Read the model definition and answer for the solid it produces. Units are mm, in the model's axes. Face numbers are marked on the shaded views. A direction names the side the tool comes from. Coordinates: 2 decimals unless noted, no trailing zeros. Write each loop counter-clockwise with the first axis right and the second up, starting at its lowest first coordinate (ties: lowest second). Pieces come first, ordered by that corner, then holes. Notation, with made-up numbers: (-28, -15) -> (-24, -15) arc R25 ccw to (-24, 24) -> close; hole circle Ø8 at (57, 63.25). An arc over 180 degrees is marked (long way). Answer in a Markdown table with one row per item. Add a question column.
Item 1: Straight lines are drawn through the part: line 1 (Y direction, x = 5.75, z = 0); line 2 (Y direction, x = 31.5, z = 5.25); line 3 (Z direction, x = 24, y = -5.5). For each, find the intervals that lie inside material, in ascending order. Write a range as from..to.
Item 2: Section B-B on z = 0 is taken. Write down the section's boundary in (x, y).
Item 3: Section C-C on x = 47.5 is taken. Write down the section's boundary in (y, z) (1 decimal), then the cut area to 3 significant figures.
Item 4: Given pin 1 Ø3 at (x, y) = (51, 1.5) entering from +Z; pin 2 Ø0.6 at (y, z) = (1.5, 4.5) entering from +X; pin 3 Ø1.5 at (x, y) = (61, -1.5) entering from -Z, each flat-ended and moving along its own axis, determine where each tip first touches the part or whether it passes through.
Item 5: Which of the six approach directions +Z, -Z, +X, -X, +Y, -Y give full straight-line access (tool end or side, diameter ignored) to the marked faces 1, 2 and 3?
Autodesk Inventor part; units mm, degrees
ref_plane "Work Plane1" through (56.23, 0, 0) normal (1, 0, 0) x (0, 0, -1)
ref_plane "YZ Plane" through (0, 0, 0) normal (1, 0, 0) x (0, 1, 0)
ref_plane "XZ Plane" through (0, 0, 0) normal (0, 1, 0) x (-1, 0, 0)
sketch "Sketch1" plane through (0, 0, 0) normal (1, 0, 0) x (0, 1, 0)
  circle A0 centre (0, 0) radius 6.35
  line L0 (0, 0) -> (0, 6.35) construction
  line L1 (-1.5875, 6.1484) -> (-1.5875, 4.7625)
  line L2 (-1.5875, 4.7625) -> (1.5875, 4.7625)
  line L3 (1.5875, 4.7625) -> (1.5875, 6.1484)
  point P0 (0, 4.7625)
  dimension "d0" = 12.7
  dimension "d2" = 1.5875
  dimension "d3" = 3.175
extrude "Extrusion1" add sketch "Sketch1" along normal blind 38.1
sketch "Sketch2" plane through (38.1, 0, 0) normal (1, 0, 0) x (0, 0, -1)
  circle A0 centre (0, 0) radius 6.35
  circle A1 centre (0, 0) radius 4.7625
  dimension "d6" = 9.525
extrude "Extrusion2" add sketch "Sketch2" along normal blind 24.13 contours A1
extrude "Extrusion3" cut sketch "Sketch1" along normal blind 34.925 contours L3 L2 L1 A0 picked at (0.1781, 5.2842)
fillet "Fillet1" radius 1.5875 2 edges at (34.925, 1.5875, 5.4554) (34.925, -1.5875, 5.4554)
chamfer "Chamfer1" distance 1.27 distance2 2.54 1 edges at (0, 0, -6.35) measured on face at (25.4, -3.3725, 5.3804)
sketch "Sketch3" plane through (0, 0, 0) normal (-1, 0, 0) x (0, 0, 1)
  circle A0 centre (0, 0) radius 3.81
  circle A1 centre (0, 0) radius 2.3495
  dimension "d16" = 4.699
extrude "Extrusion4" cut sketch "Sketch3" against normal blind 12.7 contours A1
thread "Thread1"
sketch "Sketch4" plane through (62.23, 0, 0) normal (1, 0, 0) x (0, 0, -1)
  circle A0 centre (0, 0) radius 4.7625
  line L0 (-3.5498, -3.175) -> (-3.5498, 3.175)
  line L1 (3.5498, -3.175) -> (3.5498, 3.175)
  dimension "d24" = 6.35
extrude "Extrusion5" cut sketch "Sketch4" against normal blind 5 contours A0 L1 | L0 A0
ref_plane "Work Plane1" through (56.23, 0, 0) normal (1, 0, 0) x (0, 0, -1)
sketch "Sketch5" plane through (56.23, 0, 0) normal (1, 0, 0) x (0, 0, -1)
  circle A0 centre (0, 0) radius 4.7625
  circle A1 centre (0, 0) radius 4.2926
  dimension "d28" = 8.5852
extrude "Extrusion6" cut sketch "Sketch5" against normal blind 0.7366
properties part number "Banebots 0.5x1.5 P60 Shaft" material "Steel, Carbon"
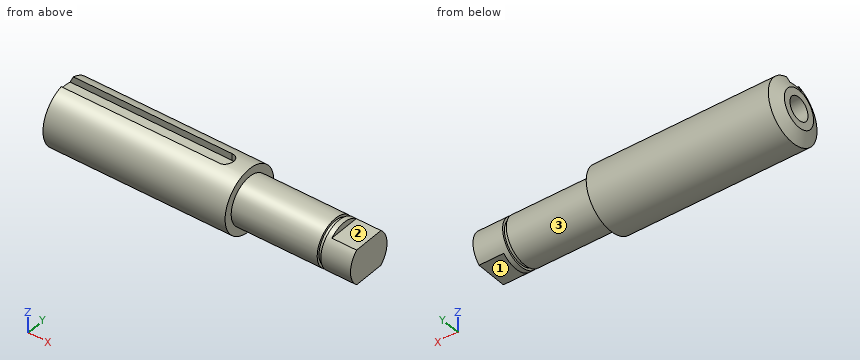
Results below:
| question | item | result |
|---|---|---|
| 1 | line 1 | y = -6.35..-2.35, 2.35..6.35 |
| 1 | line 2 | y = -3.57..-1.59, 1.59..3.57 |
| 1 | line 3 | z = -3.17..3.17 |
| 2 | outline | (0, -3.81) -> (1.27, -6.35) -> (38.1, -6.35) -> (38.1, -4.76) -> (55.49, -4.76) -> (55.49, -4.29) -> (56.23, -4.29) -> (56.23, -4.76) -> (62.23, -4.76) -> (62.23, 4.76) -> (56.23, 4.76) -> (56.23, 4.29) -> (55.49, 4.29) -> (55.49, 4.76) -> (38.1, 4.76) -> (38.1, 6.35) -> (1.27, 6.35) -> (0, 3.81) -> (0, 2.35) -> (12.7, 2.35) -> (12.7, -2.35) -> (0, -2.35) -> close |
| 3 | outline | circle Ø9.5 at (0, 0) |
| 3 | area | 71.3 mm2 |
| 4 | pin 1 | stops at z = 4.76 |
| 4 | pin 2 | stops at x = 57.23 |
| 4 | pin 3 | stops at z = -3.55 |
| 5 | face 1 | -Z, +X, +Y, -Y |
| 5 | face 2 | +Z, +X, +Y, -Y |
| 5 | face 3 | +X |
